```python
from build123d import *

# Parameters (mm, degrees)
SKETCH2_W               = 50.8
SKETCH2_H               = 50.8
BOSS_EXTRUDE1_DEPTH     = 24.765
SHELL1_START            = -6.731
SHELL1_OUTLINE_W        = 38.1
SHELL1_OUTLINE_H        = 38.1
SHELL1_DEPTH            = 25.146
SHELL1_2_OUTLINE_R      = 48.514
SHELL1_2_OUTLINE_W      = 38.1
SHELL1_2_OUTLINE_H      = 38.1
SHELL1_2_DEPTH          = 0.381
FILLET1_R               = 1.5875
FILLET2_R               = 1.5875
CUT_EXTRUDE1_DEPTH      = 82.445823816
CUT_EXTRUDE1_DEPTH_BACK = 82.445823816
SKETCH3_R               = 3.175


# Read off the part's stored shape, not the designer's step: Shell1
with BuildPart() as part:
    # Sketch1 → Revolve1 (revolve)
    with BuildSketch(Plane.XY, mode=Mode.PRIVATE) as revolve1_sk:
        Polygon((0, 0), (54.864, 0), (54.864, -22.86), (49.784, -22.86), (49.784, -6.731), (0, -6.731), align=None)
    revolve(revolve1_sk.sketch.rotate(Axis((0, -987.311672366, 0), (0, 1, 0)), 90), axis=Axis((0, -987.311672366, 0), (0, 1, 0)))

    # Sketch2 → Boss-Extrude1 (add)
    with BuildSketch(Plane(origin=(0, 0, 0), x_dir=(1, 0, 0), z_dir=(0, 1, 0))):
        Rectangle(SKETCH2_W, SKETCH2_H)
    extrude(amount=BOSS_EXTRUDE1_DEPTH)

    # Shell1 outline → Shell1 (cut)
    with BuildSketch(Plane(origin=(0, 0, 0), x_dir=(1, 0, 0), z_dir=(0, 1, 0)).offset(SHELL1_START)):
        Rectangle(SHELL1_OUTLINE_W, SHELL1_OUTLINE_H)
    extrude(amount=SHELL1_DEPTH, mode=Mode.SUBTRACT)

    # Shell1 2 outline → Shell1 2 (cut)
    with BuildSketch(Plane(origin=(0, 0, 0), x_dir=(1, 0, 0), z_dir=(0, 1, 0)).offset(SHELL1_START)):
        Circle(SHELL1_2_OUTLINE_R)
        Rectangle(SHELL1_2_OUTLINE_W, SHELL1_2_OUTLINE_H, mode=Mode.SUBTRACT)
    extrude(amount=SHELL1_2_DEPTH, mode=Mode.SUBTRACT)

    # Fillet1
    fillet1_edges = [part.edges().sort_by_distance(p)[0] for p in [
        (-25.4, 12.3825, -25.4),
        (-25.4, 12.3825, 25.4),
        (25.4, 12.3825, 25.4),
        (25.4, 12.3825, -25.4),
    ]]
    fillet(fillet1_edges, radius=FILLET1_R)

    # Fillet2
    fillet2_edges = [part.edges().sort_by_distance(p)[0] for p in [
        (0, 0, -25.4),
        (0, 24.765, -25.4),
        (25.4, 0, 0),
        (25.4, 24.765, 0),
        (-25.4, 24.765, 0),
        (0, 24.765, 25.4),
        (-24.935032015, 24.765, -24.935032015),
        (-24.935032015, 24.765, 24.935032015),
        (24.935032015, 24.765, 24.935032015),
        (24.935032015, 24.765, -24.935032015),
        (0, 0, 25.4),
        (-25.4, 0, 0),
        (24.935032015, 0, -24.935032015),
        (24.935032015, 0, 24.935032015),
        (-24.935032015, 0, 24.935032015),
        (-24.935032015, 0, -24.935032015),
    ]]
    fillet(fillet2_edges, radius=FILLET2_R)

    # Sketch3 → Cut-Extrude1 (cut, two sides: drawn at the far end of the back side and taken through both)
    with BuildSketch(Plane(origin=(0, 0, 0), x_dir=(1, 0, 0), z_dir=(0, 1, 0)).offset(-CUT_EXTRUDE1_DEPTH_BACK)):
        with Locations(Location((0, 0, 0), (0, 0, 270))):
            Circle(SKETCH3_R)
    extrude(amount=CUT_EXTRUDE1_DEPTH + CUT_EXTRUDE1_DEPTH_BACK, mode=Mode.SUBTRACT)


solid = part.part
```
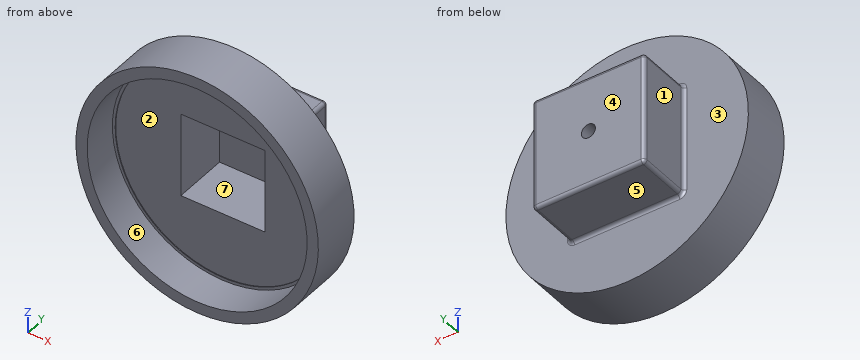
Part model, mm, in its own coordinate system. Face numbers are marked on the shaded views. A direction names the side the tool comes from. Coordinates: 2 decimals unless noted, no trailing zeros. Loops run counter-clockwise (first coordinate to the right, second up) from the corner with the lowest first, then second, coordinate; pieces in that order, holes last. Notation, with made-up numbers: (31.25, 61) - (81.25, 61) arc R20 ccw to (81.25, 91) - close; hole circle Ø3 at (16, 79). An arc over 180 degrees is marked (long way). Write item = value, one per line. Start each with the question number.
Item 1: Flat gauge pins, fed straight in: pin 1 Ø1.5 at (y, z) = (-14.5, 34) entering from -X; pin 2 Ø20 at (x, y) = (-4.5, 3) entering from +Z; pin 3 Ø4 at (y, z) = (-12, -36.5) entering from -X; pin 4 Ø6.5 at (y, z) = (12, 1.5) entering from -X. Where does each tip first touch, or does it go through?
Item 2: Wall check: L1, parallel to X at y = 21, z = 0 (3 decimals); L2, parallel to X at y = 13.5, z = -11. Give the ranges that are in metal, low to high. Write a range as from..to.
Item 3: Mould opens along Z. For the marked faces 4, 5, 6 and 7 say: released by +Z, released by -Z, zero draft, split by the parting line, or undercut.
Item 4: Cut at D-D, the plane z = 34. Give the cut face in (x, y), and give its area (3 significant figures).
Item 5: 3-axis set-ups, long thin cutter, end or side, ignore diameter. For the marked faces 1, 2 and 3: which of +Z, -Z, +X, -X, +Y, -Y reach the whole face in a straight line?
The answers:
q1.pin_1 = -43.64
q1.pin_2 = 54.86
q1.pin_3 = -42.66
q1.pin_4 = -25.4
q2.L1 = -25.4..-3.175, 3.175..25.4
q2.L2 = -25.4..-19.05, 19.05..25.4
q3.face_4 = zero draft
q3.face_5 = released by -Z
q3.face_6 = undercut
q3.face_7 = undercut
q4.outline = (-43.06, -22.86) - (-36.37, -22.86) - (-36.37, -6.73) - (-34.61, -6.73) - (-34.61, -6.35) - (34.61, -6.35) - (34.61, -6.73) - (36.37, -6.73) - (36.37, -22.86) - (43.06, -22.86) - (43.06, 0) - (-43.06, 0) - close
q4.area = 769 mm2
q5.face_1 = +Z, -Z, -X, +Y
q5.face_2 = -Y
q5.face_3 = +Y
